Geometry: final body of the model. Coordinates: model frame, mm. A direction names the side the tool comes from. Give positions to 0.01 mm unless a question says otherwise; leave off trailing zeros. Loops run counter-clockwise (first coordinate to the right, second up) from the corner with the lowest first, then second, coordinate; pieces in that order, holes last. Notation, with made-up numbers: (48.25, 78) - (87.25, 78) arc R23 cw to (87.25, 90) - close; hole circle Ø11 at (76.25, 36). An arc over 180 degrees is marked (long way). Use one line per item in the form item = value.
```python
from build123d import *

# Parameters (mm, degrees)
FILLET1_R          = 1
SKETCH2_R          = 1.5
CUT_EXTRUDE1_DEPTH = 3


with BuildPart() as part:
    # Sketch1 → Revolve1 (revolve)
    with BuildSketch(Plane.XY):
        Polygon((2, 0), (2, 4), (0, 4), (0, 10), (7, 10), (7, 7), (4, 7), (4, 0), align=None)
    revolve(axis=Axis((0, 4, 0), (0, 1, 0)))

    # Fillet1
    fillet1_edges = [part.edges().sort_by_distance(p)[0] for p in [
        (-4, 7, 0),
    ]]
    fillet(fillet1_edges, radius=FILLET1_R)

    # Sketch2 → Cut-Extrude1 (cut)
    with BuildSketch(Plane(origin=(0, 10, 0), x_dir=(1, 0, 0), z_dir=(0, 1, 0))):
        with Locations((0, 2.5)):
            Circle(SKETCH2_R)
        with Locations((0, -2.5)):
            Circle(SKETCH2_R)
    extrude(amount=-CUT_EXTRUDE1_DEPTH, mode=Mode.SUBTRACT)


solid = part.part
```
(1) Cut plane A-A (x = 0). Return the cut outline in (y, z).
Solution:
outline = (0, -4) - (6, -4) arc R1 cw to (7, -5) - (7, -7) - (10, -7) - (10, -4) - (7, -4) - (7, -1) - (10, -1) - (10, 1) - (7, 1) - (7, 4) - (10, 4) - (10, 7) - (7, 7) - (7, 5) arc R1 cw to (6, 4) - (0, 4) - (0, 2) - (4, 2) - (4, -2) - (0, -2) - close
(2) Cut plane C-C (y = 3). Return the cut outline in (x, z).
Solution:
outline = circle Ø8 at (0, 0); hole circle Ø4 at (0, 0)
(3) Cut plane D-D (y = 5.75). Return the cut outline in (x, z).
Solution:
outline = circle Ø8 at (0, 0)
(4) Material intervals for L1, parallel to Z at x = 0, y = 8; L2, parallel to Z at x = 0, y = 2, sorted ascending. Write a range as from..to.
Solution:
L1 = -7..-4, -1..1, 4..7
L2 = -4..-2, 2..4
(5) Pull-direction query (X, two-part tool) for faces 4 (the face through (-2, 0, 1)), 5 (the face through (0, 4, 0)), 6 (the face through (-0.867, 2.958, 3.905)); classes: released by +X, released by -X, zero draft, split by the parting line, or undercut.
Solution:
face_4 = zero draft
face_5 = undercut
face_6 = split by the parting line
(6) Pin query (flat end, axial travel): P1, Ø1.8, axis at x = 0, z = 2.5, coming from the -Y side; P2, Ø5, axis at y = 5, z = -5.5, coming from the -X side; P3, Ø0.9, axis at x = -0.5, z = 2, coming from the +Y side; P4, Ø1, axis at y = 4.5, z = 2.5, coming from the -X side. Return the tip coordinate at first contact, or that it passes through.
Solution:
P1 = 0
P2 = -5.74
P3 = 7
P4 = -3.46
(7) Access query for faces 1 (the face through (-2, 7, -5)), 2 (the face through (6.466, 8.479, 2.681)), 3 (the face through (0, 7, -3)). Directions: +Z, -Z, +X, -X, +Y, -Y. A direction counts if a zero-diameter tool reaches every point of the face in a straight line with its end or side. Return the directions, or none.
Solution:
face_1 = -Y
face_2 = +Y, -Y
face_3 = +Y
(8) Cut plane B-B (z = 0). Return the cut outline in (x, y), plus the area to 3 significant figures.
Solution:
outline = (-7, 7) - (-5, 7) arc R1 cw to (-4, 6) - (-4, 0) - (-2, 0) - (-2, 4) - (2, 4) - (2, 0) - (4, 0) - (4, 6) arc R1 cw to (5, 7) - (7, 7) - (7, 10) - (-7, 10) - close
area = 82.4 mm2
